Part print with two shaded views. Sizes in mm from the minimum x, y, z corner. A direction names the side the tool comes from. Round coordinates to 2 decimals unless told otherwise and drop trailing zeros. Use a Markdown table: item, result. Add a question column.
Item 1: Probe L1, parallel to Z at x = 27, y = 0.6; L2, parallel to Z at x = 12.7, y = 1.85 (1 decimal); L3, parallel to Z at x = 28, y = 2.1. List the from-to ranges inside material, lowest first.
Item 2: 3-axis set-ups, long thin cutter, end or side, ignore diameter. For the marked faces 1 and 2: which of +Z, -Z, +X, -X, +Y, -Y reach the whole face in a straight line?
Item 3: Pin check, flat tips, straight feed: pin 1 (12 mm diameter, centred on x = 14, z = 4, fed in from -Y); pin 2 (1.5 mm diameter, centred on y = 2, z = 9, fed in from +X); pin 3 (1.6 mm diameter, centred on x = 23.5, y = 2, fed in from -Z). Stop position of each tip, or through.
Item 4: Slice it at C-C, the plane y = 2.8. State how many separate pieces and enclosed holes the cut face has, plus the area to 3 significant figures.
Item 5: Two-plate mould, pull along X, no slides. Class the marked faces 3, 4 and 5: released by +X, released by -X, zero draft, split by the parting line, or undercut.
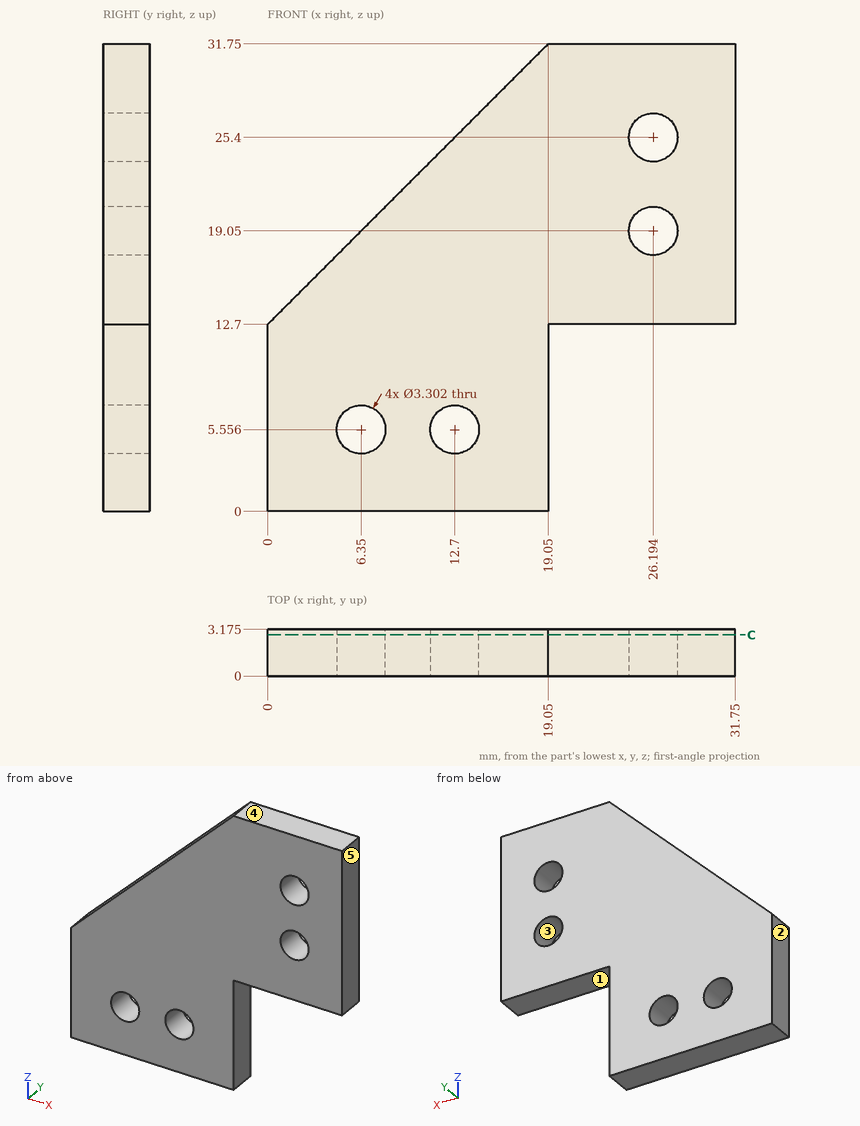
Check sheet entries:
| question | item | result |
|---|---|---|
| 1 | L1 | 12.7 to 17.61, 20.49 to 23.96, 26.84 to 31.75 |
| 1 | L2 | 0 to 3.9, 7.2 to 25.4 |
| 1 | L3 | 12.7 to 31.75 |
| 2 | face 1 | -Z, +X, +Y, -Y |
| 2 | face 2 | +Z, -Z, -X, +Y, -Y |
| 3 | pin 1 | y = 0 |
| 3 | pin 2 | x = 19.05 |
| 3 | pin 3 | z = 12.7 |
| 4 | separate pieces | 1 |
| 4 | enclosed holes | 4 |
| 4 | area | 631 mm2 |
| 5 | face 3 | undercut |
| 5 | face 4 | zero draft |
| 5 | face 5 | released by +X |
